For this review, take the finished solid that the model builds, in its own axes (mm). A direction names the side the tool comes from. Give positions to 0.01 mm unless a question says otherwise; leave off trailing zeros. Loops run counter-clockwise (first coordinate to the right, second up) from the corner with the lowest first, then second, coordinate; pieces in that order, holes last. Notation, with made-up numbers: (33.25, 32) - (78.25, 32) arc R24 cw to (78.25, 67) - close; hole circle Ø4 at (5, -15.75). An arc over 180 degrees is marked (long way). Put each result on its own line as item: value. Start each with the question number.
from build123d import *

# Parameters (mm, degrees)
EXTRUDE_1_DEPTH     = 3
FILLET_1_R          = 4
SKETCH_2_R          = 1.6
CUT_EXTRUDE_1_DEPTH = 3
SKETCH_3_R          = 2.8
CUT_EXTRUDE_2_DEPTH = 1.2
SKETCH_4_W          = 15
SKETCH_4_H          = 43
EXTRUDE_2_DEPTH     = 5
FILLET_2_R          = 1
SKETCH_5_W          = 21.917819233
SKETCH_5_H          = 11.553011577
CUT_EXTRUDE_3_DEPTH = 10


with BuildPart() as part:
    # 草图1 → 凸台-拉伸1 (new body)
    with BuildSketch(Plane(origin=(0, 0, 0), x_dir=(1, 0, 0), z_dir=(0, 1, 0))):
        Polygon((-38.5, -21.5), (38.5, -21.5), (38.5, -29.5), (46.5, -29.5), (46.5, -21.5), (46.5, 21.5), (46.5, 29.5), (38.5, 29.5), (38.5, 21.5), (-38.5, 21.5), (-38.5, 29.5), (-46.5, 29.5), (-46.5, 21.5), (-46.5, -21.5), (-46.5, -29.5), (-38.5, -29.5), align=None)
    extrude(amount=EXTRUDE_1_DEPTH)

    # 圆角1
    fillet_1_edges = [part.edges().sort_by_distance(p)[0] for p in [
        (38.5, 1.5, 29.5),
        (46.5, 1.5, 29.5),
        (-46.5, 1.5, 29.5),
        (-38.5, 1.5, 29.5),
        (-46.5, 1.5, -29.5),
        (-38.5, 1.5, -29.5),
        (38.5, 1.5, -29.5),
        (46.5, 1.5, -29.5),
    ]]
    fillet(fillet_1_edges, radius=FILLET_1_R - 0.0001)  # a hair under: the kernel refuses the full size

    # 草图2 → 切除-拉伸1 (cut)
    with BuildSketch(Plane.XZ):
        with Locations(Location((42.5, 25.5, 0), (0, 0, 270))):
            Circle(SKETCH_2_R)
        with Locations(Location((42.5, -25.5, 0), (0, 0, 90))):
            Circle(SKETCH_2_R)
        with Locations(Location((-42.5, -25.5, 0), (0, 0, 270))):
            Circle(SKETCH_2_R)
        with Locations(Location((-42.5, 25.5, 0), (0, 0, 90))):
            Circle(SKETCH_2_R)
    extrude(amount=-CUT_EXTRUDE_1_DEPTH, mode=Mode.SUBTRACT)

    # 草图3 → 切除-拉伸2 (cut)
    with BuildSketch(Plane.XZ):
        with Locations(Location((-42.5, 25.5, 0), (0, 0, 90))):
            Circle(SKETCH_3_R)
        with Locations(Location((42.5, 25.5, 0), (0, 0, 270))):
            Circle(SKETCH_3_R)
        with Locations(Location((42.5, -25.5, 0), (0, 0, 90))):
            Circle(SKETCH_3_R)
        with Locations(Location((-42.5, -25.5, 0), (0, 0, 270))):
            Circle(SKETCH_3_R)
    extrude(amount=-CUT_EXTRUDE_2_DEPTH, mode=Mode.SUBTRACT)

    # 草图4 → 凸台-拉伸2 (add)
    with BuildSketch(Plane(origin=(0, 3, 0), x_dir=(1, 0, 0), z_dir=(0, 1, 0))):
        with Locations((-39, 0)):
            Rectangle(SKETCH_4_W, SKETCH_4_H)
    extrude(amount=EXTRUDE_2_DEPTH)

    # 圆角2
    fillet_2_edges = [part.edges().sort_by_distance(p)[0] for p in [
        (-31.5, 5.5, 21.5),
        (-31.5, 5.5, -21.5),
        (-46.5, 5.5, -21.5),
        (-46.5, 5.5, 21.5),
        (-31.5, 8, 0),
        (-39, 8, -21.5),
        (-46.5, 8, 0),
        (-39, 8, 21.5),
    ]]
    fillet(fillet_2_edges, radius=FILLET_2_R)

    # 草图5 → 切除-拉伸3 (cut)
    with BuildSketch(Plane.XZ):
        with Locations((42.014050272, -27.276505788)):
            Rectangle(SKETCH_5_W, SKETCH_5_H)
    extrude(amount=-CUT_EXTRUDE_3_DEPTH, mode=Mode.SUBTRACT)


solid = part.part
1) Take a section at C-C on x = 7. State the section outline as (y, z) points, and give its area (3 significant figures).
2) Take a section at B-B on y = 4.5. State the section outline as (x, z) points.
3) Wall thickness on probe 1 along X at (y, z) = (1.6, 25.5); probe 2 along X at (y, z) = (0.8, 25.5); probe 3 along Y at (x, z) = (-18.5, -21): over which ranges is each line inside the solid? List them lowest first.
4) Mouldability with a two-part tool opening along X and no side actions: class faces 1 (the cylindrical face through (-39.641, 1.521, -28.297)), 2 (the cylindrical face through (40.796, 0.592, 27.722)), 3 (the flat face through (0, 2, -21.5)) as released by +X, released by -X, zero draft, split by the parting line, or undercut.
5) Machinability: for faces 4 (the flat face through (41, 1.2, 24)), 5 (the flat face through (6, 3, -2)), 6 (the flat face through (-38.5, 1, -23)), 7 (the cylindrical face through (39.641, 1.521, 28.297)), which of the approach directions +Z, -Z, +X, -X, +Y, -Y give a long, thin tool a straight path to every point of the face, cutting with its end or side? Answer none if there is none.
6) Insertion check: P1, Ø0.9, axis at y = 2, z = -24, coming from the +X side; P2, Ø8, axis at x = 32.5, z = 12, coming from the +Y side; P3, Ø3, axis at x = -42.5, z = 25.5, coming from the +Y side (3 decimals); P4, Ø4, axis at y = 6.5, z = -9, coming from the +X side. Each pin has a flat end and moves straight along its axis. Give the tip position at first contact, or say it passes through.
7) Take a section at A-A on z = 10.5. State the section outline as (x, y) points.
Answers follow:
1. outline: (0, -21.5) - (3, -21.5) - (3, 21.5) - (0, 21.5) - close
1. area: 129 mm2
2. outline: (-46.5, -20.5) arc R1 ccw to (-45.5, -21.5) - (-32.5, -21.5) arc R1 ccw to (-31.5, -20.5) - (-31.5, 20.5) arc R1 ccw to (-32.5, 21.5) - (-45.5, 21.5) arc R1 ccw to (-46.5, 20.5) - close
3. probe 1: -46.5 to -44.1, -40.9 to -38.5, 38.5 to 40.9, 44.1 to 46.5
3. probe 2: -46.5 to -45.3, -39.7 to -38.5, 38.5 to 39.7, 45.3 to 46.5
3. probe 3: 0 to 3
4. face 1: released by +X
4. face 2: undercut
4. face 3: zero draft
5. face 4: -Y
5. face 5: +Z, -Z, +X, +Y
5. face 6: -Z, +X, +Y, -Y
5. face 7: +Z, +Y, -Y
6. P1: x = -38.5
6. P2: y = 3
6. P3: through
6. P4: x = -31.5
7. outline: (-46.5, 0) - (46.5, 0) - (46.5, 3) - (-31.5, 3) - (-31.5, 7) arc R1 ccw to (-32.5, 8) - (-45.5, 8) arc R1 ccw to (-46.5, 7) - close
